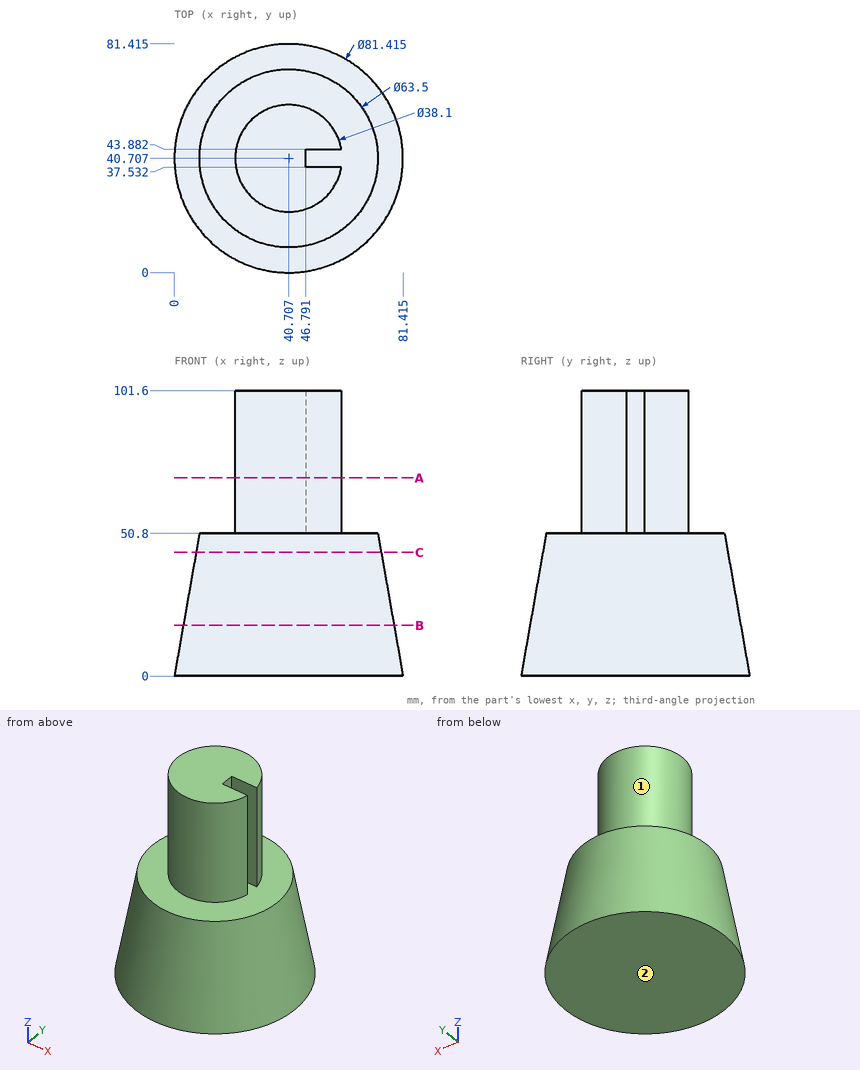
Check sheet for the drawn part. Datum: minimum x, y, z corner. Units: mm. A direction names the side the tool comes from. Round coordinates to 2 decimals unless told otherwise and drop trailing zeros. Order: outer loops, then holes, each group sorted by start corner. A loop starts at its lowest first (then second) coordinate and runs counter-clockwise, first axis right, second up.
1. Section check B-B on z = 18. Record the cut outline in (x, y), then the cut area to 3 significant figures.
Final values:
outline: circle Ø75.07 at (40.71, 40.71)
area: 4,430 mm2
2. Access from +Z, -Z, +X, -X, +Y, -Y to the whole of each face (thin tool, end or side, straight path). Record for the marked faces 1 and 2.
Final values:
face 1: +Z
face 2: -Z, +X, -X, +Y, -Y
3. Go/stop test with flat-tipped pins: P1, Ø2, axis at x = 9.5, z = 15, coming from the +Y side (1 decimal); P2, Ø4, axis at x = 53.5, z = 72.5, coming from the +Y side (1 decimal); P3, Ø1.5, axis at y = 18.5, z = 40.5, coming from the -X side. Record where each tip stops, or that it passes through.
Final values:
P1: stops at y = 63.9
P2: stops at y = 56.4
P3: stops at x = 14.87
4. Section check C-C on z = 44. Record the cut outline in (x, y), then the cut area to 3 significant figures.
Final values:
outline: circle Ø65.9 at (40.71, 40.71)
area: 3,410 mm2
5. Section check A-A on z = 70.5. Record the cut outline in (x, y), then the cut area to 3 significant figures.
Final values:
outline: (46.79, 37.53) - (46.79, 43.88) - (59.49, 43.88) arc R19.05 ccw (long way) to (59.49, 37.53) - close
area: 1,060 mm2
6. Thickness scan on L1, parallel to Z at x = 24.5, y = 56.5; L2, parallel to Y at x = 17, z = 11 (1 decimal); L3, parallel to X at y = 49.5, z = 84.5. Record the ranges inside material, lowest first.
Final values:
L1: z = 0 to 50.8
L2: y = 10 to 71.4
L3: x = 23.81 to 57.61
